```python
from build123d import *

# Parameters (mm, degrees)
F0_R     = 2.3
F1_DEPTH = 4


with BuildPart() as f1:
    # F0 (on Front) → F1 (new body)
    with BuildSketch(Plane.XZ):
        with BuildLine():
            Line((26.729051, 35.495812), (-65.270949, 35.495812))
            ThreePointArc((-65.270949, 35.495812), (-67.39227, 34.617132), (-68.270949, 32.495812))
            Line((-68.270949, 32.495812), (-68.270949, 29.495812))
            ThreePointArc((-68.270949, 29.495812), (-67.39227, 27.374491), (-65.270949, 26.495812))
            Line((-65.270949, 26.495812), (26.729051, 26.495812))
            ThreePointArc((26.729051, 26.495812), (28.850371, 27.374491), (29.729051, 29.495812))
            Line((29.729051, 29.495812), (29.729051, 32.495812))
            ThreePointArc((29.729051, 32.495812), (28.850371, 34.617132), (26.729051, 35.495812))
        make_face()
        with Locations((-58.952514, 30.995812)):
            Circle(F0_R, mode=Mode.SUBTRACT)
    extrude(amount=F1_DEPTH)


solid = f1.part
```
Geometry: final body of the model. Coordinates: model frame, mm. Round coordinates to 2 decimals unless told otherwise and drop trailing zeros. Loops run counter-clockwise (first coordinate to the right, second up) from the corner with the lowest first, then second, coordinate; pieces in that order, holes last. Notation, with made-up numbers: (-13.75, -35.5) -> (30.25, -35.5) arc R29 ccw to (30.25, -3.5) -> close; hole circle Ø7 at (9.5, 20.5). An arc over 180 degrees is marked (long way). Use one line per item in the form item = value. Start each with the question number.
1) Section A-A on y = -2.4. Output: boundary loops of the cut face in (x, z).
2) Line query: L1, parallel to X at y = -0.9, z = 31; L2, parallel to Z at x = -59, y = -3.7; L3, parallel to X at y = -2.95, z = 29.5. Output: solid intervals per line, ascending.
3) First-contact query: P1, Ø1, axis at y = -1.5, z = 28.5, coming from the -X side. Flat tip, straight axial feed; report the tip coordinate or a pass-through.
4) Draft query along X for faces 1 (the flat face through (-19, -2, 35.496)), 2 (the cylindrical face through (28.827, -1.972, 27.351)), 3 (the cylindrical face through (-56.76, -1.97, 31.69)). Return one class per face: released by +X, released by -X, zero draft, split by the parting line, or undercut.
Response:
q1.outline = (-68.27, 29.5) arc R3 ccw to (-65.27, 26.5) -> (26.73, 26.5) arc R3 ccw to (29.73, 29.5) -> (29.73, 32.5) arc R3 ccw to (26.73, 35.5) -> (-65.27, 35.5) arc R3 ccw to (-68.27, 32.5) -> close; hole circle Ø4.6 at (-58.95, 31)
q2.L1 = -68.27 to -61.25, -56.65 to 29.73
q2.L2 = 26.5 to 28.7, 33.3 to 35.5
q2.L3 = -68.27 to -60.7, -57.21 to 29.73
q3.P1 = -68.23
q4.face_1 = zero draft
q4.face_2 = released by +X
q4.face_3 = undercut
